Source: CAD feature listing. Evaluate the final solid. Frame: model axes, mm. Face numbers are marked on the shaded views. A direction names the side the tool comes from. Give positions to 0.01 mm unless a question says otherwise; leave off trailing zeros. Order: outer loops, then holes, each group sorted by start corner. A loop starts at its lowest first (then second) coordinate and runs counter-clockwise, first axis right, second up. Notation, with made-up numbers: (-7, 6.5) - (5, 6.5) arc R29 ccw to (5, 38.5) - close; hole circle Ø9 at (4, 82). An arc over 180 degrees is marked (long way). Write each question's results on one line, items separated by ' | '. Start each with the question number.
Item 1: Section C-C on z = -1.5. Output: boundary loops of the cut face in (x, y).
Item 2: Contact query for flat-ended pins moving along their axis: pin 1 Ø7.5 at (y, z) = (-40.5, -20.5) entering from +X; pin 2 Ø4 at (x, z) = (16.5, -15) entering from +Y; pin 3 Ø1.8 at (y, z) = (-34.5, 40) entering from +X; pin 4 Ø12.5 at (y, z) = (-36, -28.5) entering from -X. Output: stop coordinate, or through.
Item 3: Line query: line 1 along X through (y, z) = (-35.5, -19.5); line 2 along X through (y, z) = (-42, -36); line 3 along Y through (x, z) = (-41.5, -35). Output: solid intervals per line, ascending.
Item 4: Set-up query: the marked faces 1, 2, 3, 4 and 5. Return all of +Z, -Z, +X, -X, +Y, -Y with unobstructed straight access to the full face (end or side cutting, diameter ignored); none if empty.
Item 5: Section A-A on y = -36.5. State how many separate pieces and enclosed holes the cut face has, and give its area (3 significant figures).
Item 6: Section B-B on x = 18. Output: boundary loops of the cut face in (y, z).
```python
from build123d import *

# Parameters (mm, degrees)
F0_W     = 116.8491393328
F0_H     = 107.0637479424
F1_DEPTH = 25.4
F3_DEPTH = 25.4
F4_W     = 27.6406439953
F4_H     = 4.6218410134
F4_W_2   = 4.8651071265
F4_H_2   = 17.4579061568
F5_DEPTH = 25.4
F6_W     = 18.0926499888
F6_H     = 6.1099603772
F6_W_2   = 4.5143677853
F6_H_2   = 20.0416818261
F7_DEPTH = 25.4
F9_DEPTH = 25.4


with BuildPart() as f1:
    # F0 (on Front) → F1 (new body)
    with BuildSketch(Plane.XZ):
        Rectangle(F0_W, F0_H)
    extrude(amount=F1_DEPTH)

    # F2 (on face) → F3 (join)
    with BuildSketch(Plane.XZ.offset(25.4)):
        with BuildLine():
            add(Edge.make_bspline(
                [(-17.5561513752, 37.9903614521), (-24.953283017, 39.9782557098), (-42.8097815631, 44.7769848175), (-5.2901499603, 6.2827135922), (-35.8809845375, 7.4254009752), (-36.5513302386, 6.9073382765)],
                knots=[0, 0, 0, 0, 0.2732261888, 0.6595614733, 0.9545192624, 0.9545192624, 0.9545192624, 0.9545192624], degree=3))
            Line((-17.5561513752, 37.9903614521), (-17.5561513752, 44.0342836082))
            add(Edge.make_bspline(
                [(-17.5561513752, 44.0342836082), (-25.1543140232, 45.4079732221), (-39.6679355854, 48.0319248434), (-33.5640639258, 29.0982633355), (-16.0725558292, 11.0812579949), (-30.0093521692, 13.8591155064), (-36.5513302386, 15.1630509645)],
                knots=[0, 0, 0, 0, 0.2630540698, 0.502472426, 0.7664589194, 1, 1, 1, 1], degree=3))
            Line((-36.5513302386, 15.1630509645), (-36.5513302386, 6.9073382765))
        make_face()
    extrude(amount=F3_DEPTH)

    # F4 (on Front) → F5 (join)
    with BuildSketch(Plane.XZ):
        with Locations((2.0862433594, 40.473267436)):
            Rectangle(F4_W, F4_H)
        with BuildLine():
            add(Edge.make_bspline(
                [(2.4325535633, 20.6712316722), (3.4411130615, 16.0815352254), (5.5878055269, 6.3124865987), (-5.9730380011, 6.1934700271), (-12.1023636311, 6.1303698458)],
                knots=[0, 0, 0, 0, 0.4698202069, 1, 1, 1, 1], degree=3))
            Line((2.4325535633, 20.6712316722), (-2.4325535633, 20.6712316722))
            add(Edge.make_bspline(
                [(-12.1023636311, 12.2731719166), (-8.5431457012, 11.5565891098), (-1.4804466234, 10.1346450682), (-2.1168587101, 17.1775630293), (-2.4325535633, 20.6712316722)],
                knots=[0, 0, 0, 0, 0.5039458557, 1, 1, 1, 1], degree=3))
            Line((-12.1023636311, 12.2731719166), (-12.1023636311, 6.1303698458))
        make_face()
        with Locations((0, 29.4001847506)):
            Rectangle(F4_W_2, F4_H_2)
    extrude(amount=F5_DEPTH)

    # F6 (on face) → F7 (join)
    with BuildSketch(Plane.XZ.offset(25.4)):
        with Locations((-2.7509038337, 41.0453416407)):
            Rectangle(F6_W, F6_H)
        with Locations((-2.7444071602, 27.790505439)):
            Rectangle(F6_W_2, F6_H_2)
        with BuildLine():
            Line((-0.4872232676, 17.769664526), (-5.0015910529, 17.769664526))
            add(Edge.make_bspline(
                [(-11.7972288281, 10.6488130987), (-7.936658053, 8.5440484941), (-0.0090792572, 4.2219706922), (-3.3087786344, 13.1760440597), (-5.0015910529, 17.769664526)],
                knots=[0, 0, 0, 0, 0.4869798049, 1, 1, 1, 1], degree=3))
            Line((-11.7972288281, 10.6488130987), (-11.7972288281, 7.4829496443))
            add(Edge.make_bspline(
                [(-0.4872232676, 17.769664526), (0.7792555131, 11.7849451432), (3.2481003716, 0.1184696339), (-6.8697011613, 5.0709931812), (-11.7972288281, 7.4829496443)],
                knots=[0, 0, 0, 0, 0.5129843523, 1, 1, 1, 1], degree=3))
        make_face()
    extrude(amount=F7_DEPTH)

    # F8 (on face) → F9 (join)
    with BuildSketch(Plane.XZ.offset(25.4)):
        Polygon((-29.6439938247, -7.7707557939), (-37.9903614521, -7.7707557939), (-37.9903614521, -39.1415841877), (-33.3854667842, -39.1415841877), (-33.3854667842, -14.3902888522), (-29.6439938247, -14.3902888522), (-25.9025190026, -23.312266916), (-21.0098195821, -14.3902888522), (-17.9941952229, -14.3902888522), (-17.9941952229, -38.7041904032), (-15.2537059039, -39.1415841877), (-15.2537059039, -7.7707557939), (-21.0098195821, -7.7707557939), (-25.9025190026, -17.8439561278), align=None)
        Polygon((0, -14.2407007515), (0, -7.0455572568), (-4.40659374, -7.0455572568), (-4.40659374, -40.8627316356), (0, -40.8627316356), align=None)
        Polygon((9.408085607, -37.5529676676), (0, -7.0455572568), (0, -14.2407007515), (9.408085607, -40.1432216167), align=None)
        Polygon((9.408085607, -7.7650714666), (9.408085607, -37.5529676676), (9.408085607, -40.1432216167), (13.7251708657, -40.1432216167), (13.7251708657, -7.7650714666), align=None)
    extrude(amount=F9_DEPTH)


solid = f1.part
```
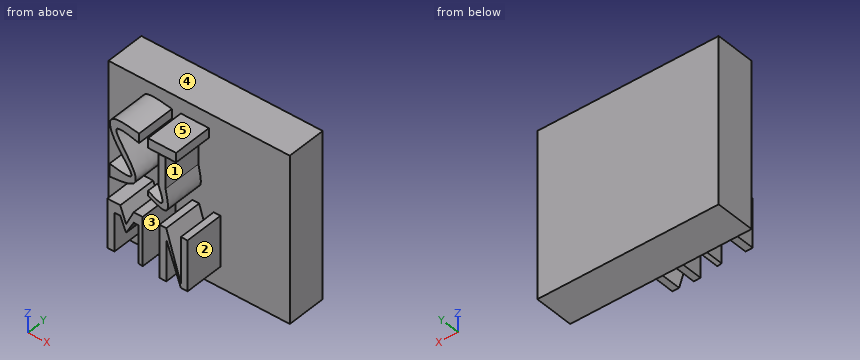
Evaluation:
1) outline: (-58.42, -25.4) - (58.42, -25.4) - (58.42, 0) - (-58.42, 0) - close
2) pin 1: stops at x = 13.73 | pin 2: stops at y = 0 | pin 3: stops at x = 6.3 | pin 4: stops at x = -37.99
3) line 1: x = -37.99 to -33.39, -27.5 to -23.81, -17.99 to -15.25, -4.41 to 0, 1.91 to 3.84, 9.41 to 13.73 | line 2: x = -37.99 to -33.39, -17.99 to -15.25, -4.41 to 0, 7.9 to 8.93, 9.41 to 13.73 | line 3: y = -25.4 to 0
4) face 1: +X, -Y | face 2: +Z, -Z, +X, -Y | face 3: +Z, -Z, -Y | face 4: +Z, +X, -X, +Y, -Y | face 5: +Z, +X, -Y
5) separate pieces: 5 | enclosed holes: 0 | area: 1,240 mm^2
6) outline: (-25.4, -53.53) - (0, -53.53) - (0, 53.53) - (-25.4, 53.53) - close
